Input: dimensioned drawing with shaded views. Units: mm. Origin: part minimum x, y, z. A direction names the side the tool comes from. Give positions to 0.01 mm unless a question says otherwise; leave off trailing zeros. Write each loop counter-clockwise with the first axis right and the second up, starting at its lowest first coordinate (ties: lowest second). Pieces come first, ordered by that corner, then holes. Notation, with made-up numbers: (70, -14) - (101, -14) arc R25 ccw to (101, -2) - close; hole circle Ø8 at (-4.75, 4.5). An arc over 180 degrees is marked (long way). Answer as a JSON object with one key per item and string values. Group by question number.
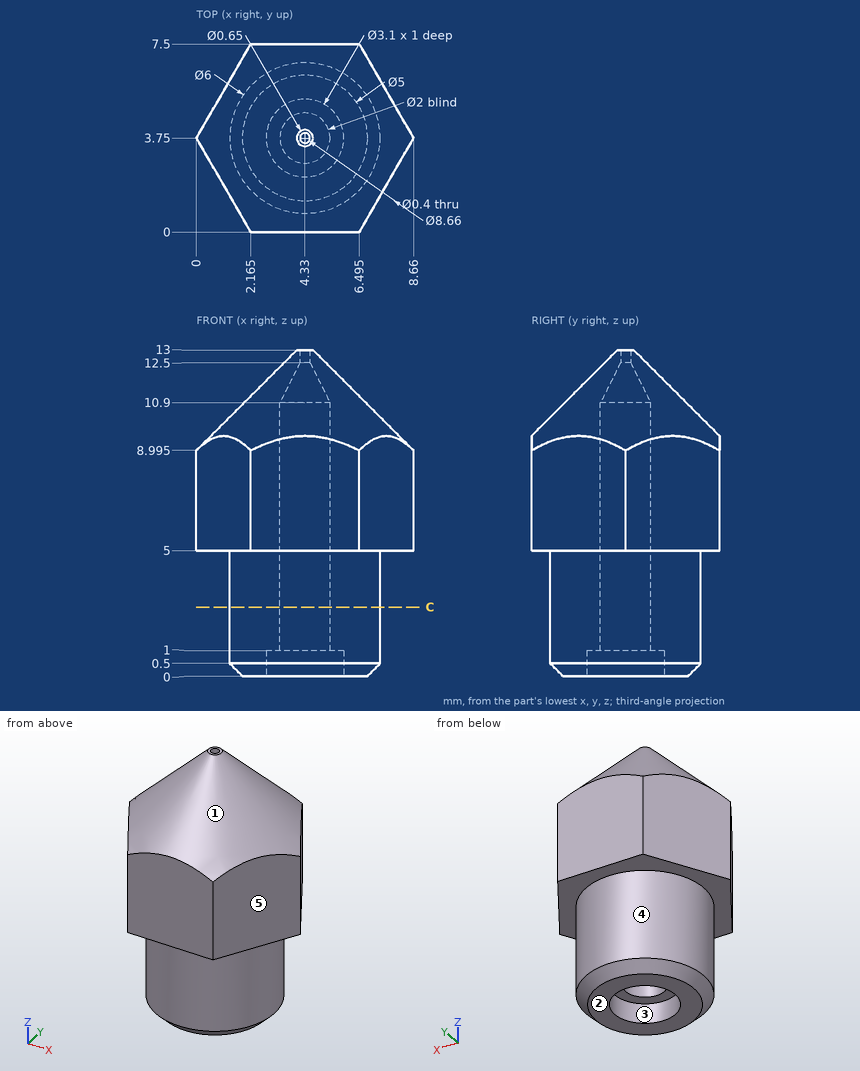
1) Pin query (flat end, axial travel): P1, Ø3, axis at x = 5.5, y = 1.5, coming from the +Z side; P2, Ø1, axis at x = 6.5, z = 10.5, coming from the -Y side; P3, Ø3, axis at y = 6.5, z = 2.5, coming from the -X side. Return the tip coordinate at first contact, or that it passes through.
2) Reachability of the marked faces 4 and 5 from +Z, -Z, +X, -X, +Y, -Y: full face, straight path, thin tool, end or side. Return the list, or none.
3) Cut plane C-C on z = 2.75. Return the cut outline in (x, y), and give its area (3 significant figures).
4) Line query: line 1 along Y through (x, z) = (3.5, 4.5); line 2 along Y through (x, z) = (3.25, 0.75); line 3 along Z through (x, y) = (3.5, 0.5). Output: solid intervals per line, ascending. Write a range as from..to.
5) Mould query, pull axis X, two halves, no side actions, for the marked faces 1, 2 and 3. Classes: +X half, -X half, draft (parallel to the pull), parting line (faces both ways), or undercut.
Filled in:
{
 "1": {"P1": "stops at z = 12.29", "P2": "stops at y = 1.12", "P3": "stops at x = 1.6"},
 "2": {"face 4": "-Z", "face 5": "+Z, -Z, +X, -Y"},
 "3": {"outline": "circle Ø6 at (4.33, 3.75); hole circle Ø2 at (4.33, 3.75)", "area": "25.1 mm²"},
 "4": {"line 1": "y = 0.87..3.19, 4.31..6.63", "line 2": "y = 0.95..2.64, 4.86..6.55", "line 3": "z = 5..9.97"},
 "5": {"face 1": "parting line", "face 2": "draft", "face 3": "undercut"}
}
